Read the model definition and answer for the solid it produces. Units are mm, in the model's axes. A direction names the side the tool comes from. Coordinates: 2 decimals unless noted, no trailing zeros. Write each loop counter-clockwise with the first axis right and the second up, starting at its lowest first coordinate (ties: lowest second). Pieces come first, ordered by that corner, then holes. Notation, with made-up numbers: (86, -28) -> (106, -28) arc R33 cw to (106, 0) -> close; hole circle Ø1 at (48.5, 42). An arc over 180 degrees is marked (long way). Write item = value, one per line. Start each with the question number.
1) Section D-D (x = 8) is taken. Determine the outline of the cut face in (y, z).
2) Section C-C (y = 3) is taken. Determine the outline of the cut face in (x, z), plus the area to 3 significant figures.
3) A tool of negligible diameter and unlimited length cuts with its end or side. For faces 1 (the face through (10.69, -6.19, 4.44)), 2 (the face through (2, 3, 9)), from which of +Z, -Z, +X, -X, +Y, -Y can it reach the whole face along a straight path? Write none if from no direction.
4) Flat-ended cylindrical pins translate along their axes: pin 1 Ø7.5 at (x, y) = (-1, -0.5) entering from -Z; pin 2 Ø4 at (x, z) = (8, 1.5) entering from +Y; pin 3 Ø3 at (x, y) = (7.5, 8.5) entering from +Z. Find the tip coordinate at first contact, or state that the pin passes through.
5) For a pull along Y with two mould halves and no side action, classify faces 3 (the face through (4.667, 7.996, 4.437)), 4 (the face through (4.57, 7.167, 9.986)), 5 (the face through (-10.69, 6.19, 4.44)), 6 (the face through (-7, 6, 9)) as released by +Y, released by -Y, zero draft, split by the parting line, or undercut.
6) Section A-A (z = 1) is taken. Determine the outline of the cut face in (x, y), plus the area to 3 significant figures.
7) Find the intervals of material crossed by line 1 along Y through (x, z) = (0, 4); line 2 along Y through (x, z) = (0, 10.35); line 3 along X through (y, z) = (0, 4.25), in increasing order. Write a range as from..to.
8) Section B-B (x = 0) is taken. Determine the outline of the cut face in (y, z).
from build123d import *

# Parameters (mm, degrees)
F0_R     = 8.5
F1_DEPTH = 9
F0_R_2   = 3.35
F2_DEPTH = 11
F3_R     = 7.5
F3_R_2   = 3.35
F4_DEPTH = 9


with BuildPart() as f1:
    # F0 (on Top) → F1 (new body)
    with BuildSketch(Plane.XY):
        with BuildLine():
            Line((-11.25833, -2), (-11.25833, -5.087327))
            ThreePointArc((-11.25833, -5.087327), (-10.699214, -6.177194), (-10.03492, -7.206336))
            Line((-10.03492, -7.206336), (-7.361216, -8.75))
            ThreePointArc((-7.361216, -8.75), (-5.111527, -7.818148), (-3.629165, -9.75))
            ThreePointArc((-3.629165, -9.75), (-3.697313, -10.267638), (-3.897114, -10.75))
            Line((-3.897114, -10.75), (-1.22341, -12.293664))
            ThreePointArc((-1.22341, -12.293664), (0, -12.354388), (1.22341, -12.293664))
            Line((1.22341, -12.293664), (3.897114, -10.75))
            ThreePointArc((3.897114, -10.75), (4.629165, -8.017949), (7.361216, -8.75))
            Line((7.361216, -8.75), (10.03492, -7.206336))
            ThreePointArc((10.03492, -7.206336), (10.699214, -6.177194), (11.25833, -5.087327))
            Line((11.25833, -5.087327), (11.25833, -2))
            ThreePointArc((11.25833, -2), (9.25833, 0), (11.25833, 2))
            Line((11.25833, 2), (11.25833, 5.087327))
            ThreePointArc((11.25833, 5.087327), (10.699214, 6.177194), (10.03492, 7.206336))
            Line((10.03492, 7.206336), (7.361216, 8.75))
            ThreePointArc((7.361216, 8.75), (4.629165, 8.017949), (3.897114, 10.75))
            Line((3.897114, 10.75), (1.22341, 12.293664))
            ThreePointArc((1.22341, 12.293664), (0, 12.354388), (-1.22341, 12.293664))
            Line((-1.22341, 12.293664), (-3.897114, 10.75))
            ThreePointArc((-3.897114, 10.75), (-3.697313, 10.267638), (-3.629165, 9.75))
            ThreePointArc((-3.629165, 9.75), (-5.111527, 7.818148), (-7.361216, 8.75))
            Line((-7.361216, 8.75), (-10.03492, 7.206336))
            ThreePointArc((-10.03492, 7.206336), (-10.699214, 6.177194), (-11.25833, 5.087327))
            Line((-11.25833, 5.087327), (-11.25833, 2))
            ThreePointArc((-11.25833, 2), (-9.844117, 1.414214), (-9.25833, 0))
            ThreePointArc((-9.25833, 0), (-9.844117, -1.414214), (-11.25833, -2))
        make_face()
        Circle(F0_R, mode=Mode.SUBTRACT)
    extrude(amount=F1_DEPTH)

    # F0 (on Top) → F2 (join)
    with BuildSketch(Plane.XY):
        Circle(F0_R)
        Circle(F0_R_2, mode=Mode.SUBTRACT)
    extrude(amount=F2_DEPTH)

    # F3 (on face) → F4 (cut)
    with BuildSketch(Plane(origin=(0, 0, 0), x_dir=(1, 0, 0), z_dir=(0, 0, -1))):
        Circle(F3_R)
        Circle(F3_R_2, mode=Mode.SUBTRACT)
    extrude(amount=-F4_DEPTH, mode=Mode.SUBTRACT)


solid = f1.part
Answer key:
q1.outline = (-8.38, 0) -> (8.38, 0) -> (8.38, 9) -> (2.87, 9) -> (2.87, 11) -> (-2.87, 11) -> (-2.87, 9) -> (-8.38, 9) -> close
q2.outline = (-11.26, 0) -> (-6.87, 0) -> (-6.87, 9) -> (-1.49, 9) -> (-1.49, 11) -> (-7.95, 11) -> (-7.95, 9) -> (-11.26, 9) -> close; (1.49, 9) -> (6.87, 9) -> (6.87, 0) -> (11.26, 0) -> (11.26, 9) -> (7.95, 9) -> (7.95, 11) -> (1.49, 11) -> close
q2.area = 105 mm^2
q3.face_1 = +Z, -Z, +X, -Y
q3.face_2 = -Z
q4.pin_1 = 9
q4.pin_2 = 8.75
q4.pin_3 = 9
q5.face_3 = undercut
q5.face_4 = split by the parting line
q5.face_5 = released by +Y
q5.face_6 = zero draft
q6.outline = (-11.26, -5.09) arc R12.35 ccw to (-10.03, -7.21) -> (-7.36, -8.75) arc R2 cw to (-3.63, -9.75) arc R2 cw to (-3.9, -10.75) -> (-1.22, -12.29) arc R12.35 ccw to (1.22, -12.29) -> (3.9, -10.75) arc R2 cw to (7.36, -8.75) -> (10.03, -7.21) arc R12.35 ccw to (11.26, -5.09) -> (11.26, -2) arc R2 cw to (11.26, 2) -> (11.26, 5.09) arc R12.35 ccw to (10.03, 7.21) -> (7.36, 8.75) arc R2 cw to (3.9, 10.75) -> (1.22, 12.29) arc R12.35 ccw to (-1.22, 12.29) -> (-3.9, 10.75) arc R2 cw to (-3.63, 9.75) arc R2 cw to (-7.36, 8.75) -> (-10.03, 7.21) arc R12.35 ccw to (-11.26, 5.09) -> (-11.26, 2) arc R2 cw to (-11.26, -2) -> close; hole circle Ø15 at (0, 0)
q6.area = 220 mm^2
q7.line_1 = -12.35..-7.5, 7.5..12.35
q7.line_2 = -8.5..-3.35, 3.35..8.5
q7.line_3 = -9.26..-7.5, 7.5..9.26
q8.outline = (-12.35, 0) -> (-7.5, 0) -> (-7.5, 9) -> (-3.35, 9) -> (-3.35, 11) -> (-8.5, 11) -> (-8.5, 9) -> (-12.35, 9) -> close; (3.35, 9) -> (7.5, 9) -> (7.5, 0) -> (12.35, 0) -> (12.35, 9) -> (8.5, 9) -> (8.5, 11) -> (3.35, 11) -> close
